Here's how the part is built. I have some questions about the finished solid (model axes, mm). A direction names the side the tool comes from. Coordinates: 2 decimals unless noted, no trailing zeros. Loops run counter-clockwise (first coordinate to the right, second up) from the corner with the lowest first, then second, coordinate; pieces in that order, holes last. Notation, with made-up numbers: M -18.5,14.25 L 9.5,14.25 A22 cw 9.5,47.25 Z; hole C -40,63.5 d5. An arc over 180 degrees is marked long. Use one line per item in the form item = value. Start each with the question number.
(1) Imagine slicing it at C-C, the plane y = 12.25. Please give me the cut outline in (x, z) (1 decimal), and give its area (3 significant figures).
(2) Please list where these lines run through material, in increasing order: L1, parallel to X at y = 3, z = 3.81; L2, parallel to Y at x = 0, z = 3.9 (3 decimals); L3, parallel to Z at x = 10.16, y = 5.25.
(3) On a 3-axis mill with a long thin cutter (end or side, diameter ignored), from which of +Z, -Z, +X, -X, +Y, -Y can I reach the whole of each face in a straight line? I mean faces 1 (the flat face through (-15, 2.54, 5)), 2 (the cylindrical face through (-0.99, 23.43, 1.72)), 3 (the cylindrical face through (-0.99, 23.43, 8.39)). Say none if no direction works.
(4) Thinking about a two-plate mould opening in Z: for faces 4 (the flat face through (15, 2.54, 5)), 5 (the flat face through (0, 8, 0)), 6 (the cylindrical face through (-11.23, 5.01, 2.14)), which applies, +Z half, -Z half, draft (parallel to the pull), parting line (faces both ways), or undercut?
(5) Imagine slicing it at B-B, the plane z = 8.5. Please give me the cut outline in (x, y) (3 decimals).
(6) Imagine slicing it at D-D, the plane x = -6.5. Please give me the cut outline in (y, z).
(7) Will these pins go through, and if not, where does the flat tip stop? P1, Ø2, axis at x = -15.5, z = 6.5, coming from the -Y side; P2, Ø1, axis at x = -9.5, z = 1.5, coming from the +Y side; P3, Ø0.8, axis at y = 1, z = 3.5, coming from the -X side.
(8) Imagine slicing it at A-A, the plane x = 0. Please give me the cut outline in (y, z) (1 decimal), and give its area (3 significant figures).
```python
from build123d import *

# Parameters (mm, degrees)
SKETCH1_R                = 7.62
BOSS_EXTRUDE1_DEPTH      = 10.16
SKETCH3_R                = 8.7376
SKETCH3_R_2              = 3.27025
BOSS_EXTRUDE2_DEPTH      = 1.5875
BOSS_EXTRUDE2_DEPTH_BACK = 1.5875
SKETCH4_R                = 1.98374
CUT_EXTRUDE1_DEPTH       = 10.16


with BuildPart() as part:
    # Sketch1 → Boss-Extrude1 (new body)
    with BuildSketch(Plane.XY):
        with BuildLine():
            Line((4.5, 4.699), (-4.5, 4.699))
            Line((-4.5, 4.699), (-4.5, 0))
            Line((-4.5, 0), (-13.97, 0))
            Line((-13.97, 0), (-13.97, 2.54))
            Line((-13.97, 2.54), (-16.51, 2.54))
            Line((-16.51, 2.54), (-16.51, 10.795))
            Line((-16.51, 10.795), (-11.43, 15.875))
            ThreePointArc((-11.43, 15.875), (0, 27.305), (11.43, 15.875))
            Line((11.43, 15.875), (16.51, 10.795))
            Line((16.51, 10.795), (16.51, 2.54))
            Line((16.51, 2.54), (13.97, 2.54))
            Line((13.97, 2.54), (13.97, 0))
            Line((13.97, 0), (4.5, 0))
            Line((4.5, 0), (4.5, 4.699))
        make_face()
        with Locations((0, 15.875)):
            Circle(SKETCH1_R, mode=Mode.SUBTRACT)
    extrude(amount=BOSS_EXTRUDE1_DEPTH)

    # Sketch3 → Boss-Extrude2 (add, two sides)
    with BuildSketch(Plane.XY.offset(5.08)) as boss_extrude2_sk:
        with Locations((0, 15.875)):
            Circle(SKETCH3_R)
        with Locations((0, 15.875)):
            Circle(SKETCH3_R_2, mode=Mode.SUBTRACT)
    extrude(amount=BOSS_EXTRUDE2_DEPTH)
    extrude(boss_extrude2_sk.sketch, amount=-BOSS_EXTRUDE2_DEPTH_BACK)

    # Sketch4 → Cut-Extrude1 (cut)
    with BuildSketch(Plane(origin=(0, 0, 0), x_dir=(-1, 0, 0), z_dir=(0, -1, 0))):
        with Locations((-10.16, -3.81)):
            Circle(SKETCH4_R)
        with Locations((10.16, -3.81)):
            Circle(SKETCH4_R)
    extrude(amount=-CUT_EXTRUDE1_DEPTH, mode=Mode.SUBTRACT)


solid = part.part
```
Answer:
q1.outline = M -15.1,0 L -6.7,0 L -6.7,3.5 L 6.7,3.5 L 6.7,0 L 15.1,0 L 15.1,10.2 L 6.7,10.2 L 6.7,6.7 L -6.7,6.7 L -6.7,10.2 L -15.1,10.2 Z
q1.area = 212 mm²
q2.L1 = -16.51 to -12.14, -8.18 to -4.5, 4.5 to 8.18, 12.14 to 16.51
q2.L2 = 4.699 to 12.605, 19.145 to 27.305
q2.L3 = 0 to 1.83, 5.79 to 10.16
q3.face_1 = +Z, -Z, -X, -Y
q3.face_2 = -Z
q3.face_3 = +Z
q4.face_4 = draft
q4.face_5 = -Z half
q4.face_6 = undercut
q5.outline = M -16.51,2.54 L -13.97,2.54 L -13.97,0 L -4.5,0 L -4.5,4.699 L 4.5,4.699 L 4.5,0 L 13.97,0 L 13.97,2.54 L 16.51,2.54 L 16.51,10.795 L 11.43,15.875 A11.43 ccw -11.43,15.875 L -16.51,10.795 Z; hole C 0,15.875 d15.24
q6.outline = M 0,0 L 11.9,0 L 11.9,3.49 L 19.85,3.49 L 19.85,0 L 25.28,0 L 25.28,10.16 L 19.85,10.16 L 19.85,6.67 L 11.9,6.67 L 11.9,10.16 L 0,10.16 Z
q7.P1 = 2.54
q7.P2 = 22.92
q7.P3 = -13.97
q8.outline = M 4.7,0 L 8.3,0 L 8.3,3.5 L 12.6,3.5 L 12.6,6.7 L 8.3,6.7 L 8.3,10.2 L 4.7,10.2 Z; M 19.1,3.5 L 23.5,3.5 L 23.5,0 L 27.3,0 L 27.3,10.2 L 23.5,10.2 L 23.5,6.7 L 19.1,6.7 Z
q8.area = 102 mm²
